Autodesk Inventor part; units mm, degrees
ref_plane "YZ Plane" through (0, 0, 0) normal (1, 0, 0) x (0, 1, 0)
ref_plane "XZ Plane" through (0, 0, 0) normal (0, 1, 0) x (-1, 0, 0)
ref_plane "XY Plane" through (0, 0, 0) normal (0, 0, 1) x (1, 0, 0)
sketch "Sketch5" plane through (0, 0, 0) normal (0, 1, 0) x (-1, 0, 0)
  line L0 (45, 30) -> (-45, 30)
  line L1 (-45, 30) -> (-45, -30)
  line L2 (-45, -30) -> (45, -30)
  line L3 (45, -30) -> (45, 30)
  point P0 (0, 0)
  point P1 (0, 30)
  point P2 (45, 0)
  dimension "d8" = 90
  dimension "d9" = 60
extrude "Extrusion5" add sketch "Sketch5" along normal blind 91.85
sketch "Sketch6" plane through (-45, 0, 30) normal (0, 0, 1) x (1, 0, 0)
  line L0 (0, 0) -> (90, 0)
  line L1 (0, 91.85) -> (90, 91.85)
  line L2 (35, 91.85) -> (55, 91.85)
  line L3 (55, 91.85) -> (55, 65.85)
  line L4 (55, 65.85) -> (35, 65.85)
  line L5 (35, 65.85) -> (35, 91.85)
  point P0 (45, 0)
  point P1 (45, 65.85)
  point P2 (45, 0)
  dimension "d12" = 26
  dimension "d13" = 20
extrude "Extrusion6" add sketch "Sketch6" along normal blind 5
chamfer "Chamfer2" distance 5 angle 45 2 edges at (10, 91.85, 32.5) (-10, 91.85, 32.5)
sketch "Sketch8" plane through (45, 0, -30) normal (0, 0, -1) x (-1, 0, 0)
  line L0 (0, 0) -> (90, 0)
  line L1 (90, 0) -> (90, 91.85)
  line L2 (0, 91.85) -> (90, 91.85)
  line L3 (0, 0) -> (0, 91.85)
  line L4 (20.5, 17) -> (20.5, 91.85)
  line L5 (45, 0) -> (45, 11.253)
  line L6 (45, 91.85) -> (45, 84.4514)
  line L7 (69.5, 91.85) -> (69.5, 17)
  line L8 (77.5, 17) -> (90, 17)
  line L9 (77.5, 17) -> (69.5, 17)
  line L10 (20.5, 17) -> (0, 17)
  point P0 (20.5, 25)
  point P1 (12.5, 17)
  point P2 (69.5, 25)
  dimension "d42" = 90
extrude "Extrusion7" cut sketch "Sketch8" against normal blind 40 contours L3 L2 L4 L10 | L8 L9 L7 L2 L1
sketch "Sketch9" plane through (45, 0, 10) normal (0, 0, -1) x (-1, 0, 0)
  circle A0 centre (10, 77) radius 5
  circle A1 centre (80, 77) radius 5
  line L0 (0, 0) -> (90, 0)
  line L1 (0, 17) -> (0, 91.85)
  circle A2 centre (10, 77) radius 10
  line L2 (0, 91.85) -> (90, 91.85)
  line L3 (45, 91.85) -> (45, 95.8754) construction
  line L4 (20.5, 91.85) -> (20.5, 17) construction
  point P0 (45, 0)
  dimension "d47" = 10
  dimension "d56" = 70
  dimension "d58" = 77
  dimension "d61" = 20
  dimension "d62" = 35
  dimension "d63" = 20.5
hole "Hole2" at (-35, 77, 10) at (35, 77, 10) direction (0, 0, 1) diameter 10.5 end through all
fillet "Fillet3" radius 6 2 edges at (34.75, 17, 10) (-34.75, 17, 10)
sketch "Sketch11" plane through (0, 0, 0) normal (0, -1, 0) x (1, 0, 0)
  line L0 (45, -30) -> (-45, -30)
  circle A0 centre (-35, -8) radius 5.25
  circle A1 centre (35, -8) radius 5.25
  circle A2 centre (-35, -8) radius 10
  line L1 (-24.5, 4) -> (-45, 4)
  point P0 (0, 0)
  dimension "d64" = 70
  dimension "d65" = 10.5
  dimension "d66" = 20
  dimension "d67" = 22
  dimension "d75" = 35
  dimension "d76" = 34
hole "Hole3" at (-35, 0, -8) at (35, 0, -8) direction (0, 1, 0) diameter 10.5 end through all
sketch "Sketch12" plane through (45, 0, 30) normal (1, 0, 0) x (0, 0, -1)
  line L0 (0, 0) -> (0, 91.85)
  line L1 (0, 0) -> (60, 0)
  line L2 (0, 0) -> (1, 0)
  line L3 (1, 0) -> (1, 63)
  line L4 (1, 63) -> (0, 63)
  line L5 (0, 63) -> (0, 0)
  point P0 (30, 0)
  dimension "d77" = 1
  dimension "d78" = 63
  dimension "d79" = 0
extrude "Extrusion8" cut sketch "Sketch12" against normal through all
sketch "Sketch13" plane through (45, 0, 10) normal (0, 0, -1) x (-1, 0, 0)
  circle A0 centre (10, 77) radius 5.25
  circle A1 centre (10, 48) radius 4
  circle A2 centre (10, 27) radius 4
  line L0 (0, 0) -> (90, 0)
  circle A3 centre (80, 77) radius 5.25
  line L1 (45, 0) -> (45, -5.7212)
  circle A4 centre (80, 48) radius 4
  circle A5 centre (80, 27) radius 4
  dimension "d82" = 27
  dimension "d83" = 70
  dimension "d84" = 8
  dimension "d85" = 48
hole "Hole4" at (35, 48, 10) at (35, 27, 10) at (-35, 48, 10) at (-35, 27, 10) direction (0, 0, 1) diameter 6.647 end through all
sketch "Sketch16" plane through (0, 0, 0) normal (0, -1, 0) x (1, 0, 0)
  line L0 (-45, 29) -> (-41, 29)
  line L1 (-45, 25) -> (-45, 29)
  line L2 (-45, 25) -> (-41, 29)
  line L3 (0, 0) -> (0, -4.4881)
  line L4 (45, 29) -> (41, 29)
  line L5 (45, 25) -> (45, 29)
  line L6 (45, 25) -> (41, 29)
  line L7 (0, 0) -> (2.8094, 0)
  line L8 (-45, -30) -> (-40, -30)
  line L9 (-45, -25) -> (-45, -30)
  line L10 (-45, -25) -> (-40, -30)
  line L11 (45, -30) -> (40, -30)
  line L12 (45, -25) -> (45, -30)
  line L13 (45, -25) -> (40, -30)
  line L14 (45, -30) -> (-45, -30)
  line L15 (45, 29) -> (45, -30)
  dimension "d96" = 4
  dimension "d97" = 4
  dimension "d100" = 5
  dimension "d101" = 5
  dimension "d102" = 5
  dimension "d103" = 5
  dimension "d104" = 4
extrude "Extrusion10" cut sketch "Sketch16" against normal up to surface (17 mm away) from surface at 0
equation "\"d62\" = 0.5 * d56"
equation "\"d102\" = d101"
equation "\"d103\" = d100"
properties part number "BC-10019-B" material "Alumínio 7075"
For this review, take the finished solid that the model builds, in its own axes (mm). A direction names the side the tool comes from. Give positions to 0.01 mm unless a question says otherwise; leave off trailing zeros. Order: outer loops, then holes, each group sorted by start corner. A loop starts at its lowest first (then second) coordinate and runs counter-clockwise, first axis right, second up. Notation, with made-up numbers: (0.25, 35.25) - (34.25, 35.25) arc R20 cw to (34.25, 62.25) - close; hole circle Ø8 at (31.5, -30.75). An arc over 180 degrees is marked (long way). Answer as a JSON object with one key per item and string values. Group by question number.
Item 1: Take a section at C-C on z = 14.5. Give the boundary of the cut face in (x, y), and give its area (3 significant figures).
Item 2: Machinability: for faces 1 (the flat face through (-10, 76, 32)), 2 (the flat face through (-43, 8, 27)), 3 (the cylindrical face through (-34.894, 18.711, 8.196)), 4 (the flat face through (35, 58, 10)), which of the approach directions +Z, -Z, +X, -X, +Y, -Y give a long, thin tool a straight path to every point of the face, cutting with its end or side? Answer none if there is none.
Item 3: Take a section at B-B on x = 35. Give the boundary of the cut face in (y, z), and give its area (3 significant figures).
Item 4: Take a section at D-D on y = 8. Give the boundary of the cut face in (x, z), and give its area (3 significant figures).
Item 5: Clearance check with flat-ended pins moving along their axes: pin 1 Ø12 at (x, y) = (-35, 77) entering from -Z; pin 2 Ø16.5 at (x, z) = (33.5, -4.5) entering from +Y; pin 3 Ø0.5 at (x, z) = (18.5, 29.5) entering from -Y. State where each tip first meets the part, or that it passes through.
Item 6: Draft analysis for pull direction X (two halves, no side actions). For faces 5 (the flat face through (-45, 35, 14)), 6 (the flat face through (32, 17, -13)), 7 (the cylindrical face through (30.57, 8.62, -10.82)), 8 (the cylindrical face through (-39.43, 8.62, -10.82)), state which applies: pulls with the +X half, pulls with the -X half, needs draft (parallel to the pull), parting line crosses it, or undercut.
Item 7: Take a section at A-A on y = 77. Give the boundary of the cut face in (x, z).
Item 8: Wall thickness on line 1 along Y through (x, z) = (-35, 14.25); line 2 along X through (y, z) = (48, 18.75); line 3 along X through (y, z) = (12.75, -8): over which ranges is each line inside the solid? List them lowest first.
Reported:
{
 "1": {"outline": "(-45, 0) - (45, 0) - (45, 91.85) - (-45, 91.85) - close; hole circle Ø10.5 at (-35, 77); hole circle Ø6.65 at (-35, 27); hole circle Ø6.65 at (-35, 48); hole circle Ø10.5 at (35, 77); hole circle Ø6.65 at (35, 27); hole circle Ø6.65 at (35, 48)", "area": "7,950 mm^2"},
 "2": {"face 1": "+Z, -X, +Y, -Y", "face 2": "+Z, -X, -Y", "face 3": "-Z, -X, +Y", "face 4": "-Z, +X, +Y"},
 "3": {"outline": "(0, -30) - (17, -30) - (17, -13.25) - (0, -13.25) - close; (0, -2.75) - (17, -2.75) - (17, 4) arc R6 cw to (23, 10) - (23.68, 10) - (23.68, 29) - (0, 29) - close; (30.32, 10) - (44.68, 10) - (44.68, 29) - (30.32, 29) - close; (51.32, 10) - (71.75, 10) - (71.75, 30) - (63, 30) - (63, 29) - (51.32, 29) - close; (82.25, 10) - (91.85, 10) - (91.85, 30) - (82.25, 30) - close", "area": "1,820 mm^2"},
 "4": {"outline": "(-45, -25) - (-40, -30) - (40, -30) - (45, -25) - (45, 25) - (41, 29) - (-41, 29) - (-45, 25) - close; hole circle Ø10.5 at (-35, -8); hole circle Ø10.5 at (35, -8)", "area": "5,100 mm^2"},
 "5": {"pin 1": "z = 10", "pin 2": "y = 17", "pin 3": "y = 63"},
 "6": {"face 5": "pulls with the -X half", "face 6": "needs draft", "face 7": "undercut", "face 8": "undercut"},
 "7": {"outline": "(-45, 10) - (-40.25, 10) - (-40.25, 30) - (-45, 30) - close; (-29.75, 10) - (-24.5, 10) - (-24.5, -30) - (24.5, -30) - (24.5, 10) - (29.75, 10) - (29.75, 30) - (10, 30) - (10, 35) - (-10, 35) - (-10, 30) - (-29.75, 30) - close; (40.25, 10) - (45, 10) - (45, 30) - (40.25, 30) - close"},
 "8": {"line 1": "0 to 23.68, 30.32 to 44.68, 51.32 to 71.75, 82.25 to 91.85", "line 2": "-45 to -38.32, -31.68 to 31.68, 38.32 to 45", "line 3": "-45 to -40.25, -29.75 to 29.75, 40.25 to 45"}
}
